from build123d import *

# Parameters (mm, degrees)
F1_DEPTH = 25.4
F3_DEPTH = 25.4
F4_R     = 12.7
F5_DEPTH = 25.4


with BuildPart() as f1:
    # F0 (on Front) → F1 (new body)
    with BuildSketch(Plane.XZ):
        Polygon((403.225, 12.7), (428.625, 12.7), (428.625, 298.45), (428.625, 323.85), (-428.625, 323.85), (-428.625, 298.45), (-428.625, 12.7), (-403.225, 12.7), (-403.225, 298.45), (-43.6594735359, 12.7), (-7.9375, 12.7), (14.2875, 12.7), (49.6461265683, 12.7), (403.225, 298.45), align=None)
        Polygon((-7.9375, 298.45), (-7.9375, 12.7), (-367.5030264641, 298.45), align=None, mode=Mode.SUBTRACT)
        Polygon((367.8663734317, 298.45), (14.2875, 12.7), (14.2875, 298.45), align=None, mode=Mode.SUBTRACT)
        Polygon((428.625, 0), (428.625, 12.7), (403.225, 12.7), (49.6461265683, 12.7), (14.2875, 12.7), (-7.9375, 12.7), (-43.6594735359, 12.7), (-403.225, 12.7), (-428.625, 12.7), (-428.625, 0), align=None)
    extrude(amount=F1_DEPTH)

    # F2 (on face) → F3 (join)
    with BuildSketch(Plane.XZ.offset(25.4)):
        Polygon((-339.725, 12.7), (-403.225, 76.2), (-403.225, 12.7), align=None)
        Polygon((403.225, 76.2), (339.725, 12.7), (403.225, 12.7), align=None)
    extrude(amount=-F3_DEPTH)

    # F4 (on Front) → F5 (join)
    with BuildSketch(Plane.XZ):
        with Locations((-302.4, 207.65)):
            Circle(F4_R)
        with Locations((302.4, 207.65)):
            Circle(F4_R)
    extrude(amount=-F5_DEPTH)


solid = f1.part
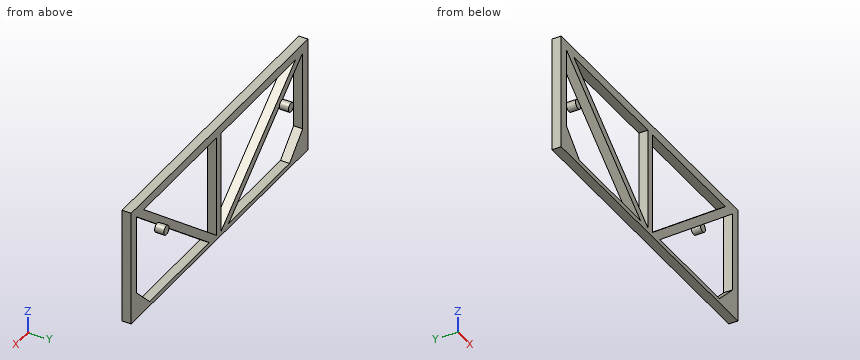
Input: part model. Units: mm. Frame: model coordinates. Coordinates: 2 decimals unless noted, no trailing zeros. Loops run counter-clockwise (first coordinate to the right, second up) from the corner with the lowest first, then second, coordinate; pieces in that order, holes last. Notation, with made-up numbers: (48.25, 39) - (99.25, 39) arc R29 ccw to (99.25, 75) - close; hole circle Ø3 at (-33, -15.5). An arc over 180 degrees is marked (long way). Answer in a Markdown table with one row per item. Add a question column.
Item 1: Section query C-C on x = -103. Return the cut outline in (y, z).
Item 2: Section query D-D on x = 121. Return the cut outline in (y, z).
Item 3: Section query B-B on z = 45. Return the cut outline in (x, y) (1 decimal), then the cut area to 3 significant figures.
Item 4: Line query: line 1 along X through (y, z) = (-20, 188) (1 decimal); line 2 along Z through (x, y) = (266.5, -12); line 3 along Z through (x, y) = (-359, -8) (3 decimals). Output: solid intervals per line, ascending. Write a range as [from, to].
Item 5: Contact query for a flat-ended pin moving along its axis: P1, Ø7.5, axis at x = -306, z = 203, coming from the -Y side. Output: stop coordinate, or through.
Item 6: Section query A-A on y = -13. State how many separate pieces and enclosed holes the cut face has, then the cut area to 3 significant figures.
Recorded:
| question | item | result |
|---|---|---|
| 1 | outline | (-25.4, 0) - (0, 0) - (0, 12.7) - (-25.4, 12.7) - close; (-25.4, 59.86) - (0, 59.86) - (0, 88.25) - (-25.4, 88.25) - close; (-25.4, 298.45) - (0, 298.45) - (0, 323.85) - (-25.4, 323.85) - close |
| 2 | outline | (-25.4, 0) - (0, 0) - (0, 12.7) - (-25.4, 12.7) - close; (-25.4, 70.37) - (0, 70.37) - (0, 98.94) - (-25.4, 98.94) - close; (-25.4, 298.45) - (0, 298.45) - (0, 323.85) - (-25.4, 323.85) - close |
| 3 | outline | (-428.6, -25.4) - (-372, -25.4) - (-372, 0) - (-428.6, 0) - close; (-84.3, -25.4) - (-48.6, -25.4) - (-48.6, 0) - (-84.3, 0) - close; (-7.9, -25.4) - (14.3, -25.4) - (14.3, 0) - (-7.9, 0) - close; (54.3, -25.4) - (89.6, -25.4) - (89.6, 0) - (54.3, 0) - close; (372, -25.4) - (428.6, -25.4) - (428.6, 0) - (372, 0) - close |
| 3 | area | 5,250 mm^2 |
| 4 | line 1 | [-428.6, -403.2], [-264.2, -228.5], [-7.9, 14.3], [231.2, 266.6], [403.2, 428.6] |
| 4 | line 2 | [0, 12.7], [187.95, 216.53], [298.45, 323.85] |
| 4 | line 3 | [0, 31.975], [263.304, 291.693], [298.45, 323.85] |
| 5 | P1 | y = 0 |
| 6 | separate pieces | 1 |
| 6 | enclosed holes | 4 |
| 6 | area | 77,900 mm^2 |
